Work out the finished part from the listing and answer in its coordinate system (mm). A direction names the side the tool comes from. Round coordinates to 2 decimals unless told otherwise and drop trailing zeros. Loops run counter-clockwise (first coordinate to the right, second up) from the corner with the lowest first, then second, coordinate; pieces in that order, holes last. Notation, with made-up numbers: M 61,51.5 L 78,51.5 A26 cw 78,74.5 Z; hole C -31,58 d9. An arc over 180 degrees is marked long. One line per item, written item: value.
```python
from build123d import *

# Parameters (mm, degrees)
BOX052_W     = 10
BOX052_H     = 17
BOX052_DEPTH = 1
BOX024_W     = 9
BOX024_H     = 1
BOX024_DEPTH = 2
BOX022_W     = 1
BOX022_H     = 16
BOX022_DEPTH = 9
BOX021_W     = 10
BOX021_H     = 1
BOX021_DEPTH = 9
BOX025_W     = 10
BOX025_H     = 17
BOX025_DEPTH = 1


with BuildPart() as box052:
    # Box052 → Box052 (new body)
    with BuildSketch(Plane(origin=(-10, 8, 0), x_dir=(1, 0, 0), z_dir=(0, 0, 1))):
        with Locations((5, 8.5)):
            Rectangle(BOX052_W, BOX052_H)
    extrude(amount=BOX052_DEPTH)


with BuildPart() as box024:
    # Box024 → Box024 (new body)
    with BuildSketch(Plane(origin=(-9, 24, 7), x_dir=(1, 0, 0), z_dir=(0, 0, 1))):
        with Locations((4.5, 0.5)):
            Rectangle(BOX024_W, BOX024_H)
    extrude(amount=BOX024_DEPTH)


with BuildPart() as box022:
    # Box022 → Box022 (new body)
    with BuildSketch(Plane(origin=(-10, 9, 0), x_dir=(1, 0, 0), z_dir=(0, 0, 1))):
        with Locations((0.5, 8)):
            Rectangle(BOX022_W, BOX022_H)
    extrude(amount=BOX022_DEPTH)


with BuildPart() as box021:
    # Box021 → Box021 (new body)
    with BuildSketch(Plane(origin=(-10, 8, 0), x_dir=(1, 0, 0), z_dir=(0, 0, 1))):
        with Locations((5, 0.5)):
            Rectangle(BOX021_W, BOX021_H)
    extrude(amount=BOX021_DEPTH)


with BuildPart() as fusion024:
    # Box025 → Box025 (new body)
    with BuildSketch(Plane(origin=(-10, 8, 9), x_dir=(1, 0, 0), z_dir=(0, 0, 1))):
        with Locations((5, 8.5)):
            Rectangle(BOX025_W, BOX025_H)
    extrude(amount=BOX025_DEPTH)

    # Fusion010: union Box024, Box022, Box021
    add(box024.part)
    add(box022.part)
    add(box021.part)


with BuildPart() as fusion024_1:
    # Fusion010 placement: moved
    add(fusion024.part.moved(Location((0, 0, 1))))

    # Fusion024: union Box052
    add(box052.part)


solid = fusion024_1.part
```
1) For faces 4 (the face through (-10, 16, 5)), 5 (the face through (-4.6, 24.5, 8)), 6 (the face through (-5, 9, 5)), determine the directions among +Z, -Z, +X, -X, +Y, -Y from which every point of the face is accessible in a straight line to the end or side of a thin tool.
Check values:
face 4: +Z, -Z, -X, +Y, -Y
face 5: +X, +Y
face 6: +X
2) The mould has two halves that part along Y. Classify faces 1 (the face through (-6, 25, 9)), 2 (the face through (-5, 17, 0)), 3 (the face through (-5, 24, 9)): +Y half, -Y half, draft (parallel to the pull), parting line (faces both ways), or undercut.
Check values:
face 1: +Y half
face 2: draft
face 3: undercut
3) Find the intervals of material crossed by probe 1 along Z at (x, y) = (-0.5, 12.25); probe 2 along Y at (x, z) = (-8, 9); probe 3 along Y at (x, z) = (-7.25, 4.75), in increasing order. Write a range as from..to.
Check values:
probe 1: 0..1, 10..11
probe 2: 8..9, 24..25
probe 3: 8..9
4) Find section A-A (x = -2.25). Give the vertices of the cut face in (y, z).
Check values:
outline: M 8,0 L 25,0 L 25,1 L 9,1 L 9,10 L 24,10 L 24,8 L 25,8 L 25,11 L 8,11 Z
5) Find section C-C (z = 5.75). Give the vertices of the cut face in (x, y).
Check values:
outline: M -10,8 L 0,8 L 0,9 L -9,9 L -9,25 L -10,25 Z
6) Each of these flat-tipped pins is pushed along its axis until it touches: pin 1 (4.5 mm diameter, centred on x = -4.5, y = 15.5, fed in from -Z); pin 2 (3 mm diameter, centred on x = -5, z = 5.5, fed in from +Y); pin 3 (1 mm diameter, centred on y = 16, z = 2.5, fed in from +X). Where does it stop, or does it pass through?
Check values:
pin 1: z = 0
pin 2: y = 9
pin 3: x = -9
7) Find section B-B (y = 19). Give the vertices of the cut face in (x, z).
Check values:
outline: M -10,0 L 0,0 L 0,1 L -9,1 L -9,10 L 0,10 L 0,11 L -10,11 Z
